Input: part model. Units: mm. Frame: model coordinates. A direction names the side the tool comes from. Give positions to 0.01 mm unless a question says otherwise; leave off trailing zeros. Write each loop counter-clockwise with the first axis right and the second up, starting at its lowest first coordinate (ties: lowest second). Pieces come first, ordered by that corner, then holes. Notation, with made-up numbers: (41, 50) -> (90, 50) arc R28 cw to (90, 73) -> close; hole circle Ø2 at (49.25, 57.5). An arc over 180 degrees is marked (long way). Answer as a JSON object with one key per item and string values. Group by question number.
Autodesk Inventor part; units mm, degrees
ref_plane "YZ Plane" through (0, 0, 0) normal (1, 0, 0) x (0, 1, 0)
ref_plane "XZ Plane" through (0, 0, 0) normal (0, 1, 0) x (-1, 0, 0)
ref_plane "XY Plane" through (0, 0, 0) normal (0, 0, 1) x (1, 0, 0)
sketch "Sketch1" plane through (0, 0, 0) normal (0, 0, 1) x (1, 0, 0)
  line L0 (0, 0) -> (0, 13.5)
  line L1 (0, 13.5) -> (36, 13.5)
  line L2 (36, 13.5) -> (36, 4.4)
  line L3 (36, 4.4) -> (40.4, 4.4)
  line L4 (40.4, 4.4) -> (40.4, 0)
  line L5 (40.4, 0) -> (0, 0)
  line L6 (0, 0) -> (68.0723, 0)
  dimension "d0" = 27
  dimension "d1" = 36
  dimension "d2" = 8.8
  dimension "d3" = 4.4
revolve "Revolution1" add sketch "Sketch1" angle 360 about axis through (0, 0, 0) along (1, 0, 0)
sketch "Sketch2" plane through (40.4, 0, 0) normal (1, 0, 0) x (0, 0, -1)
  circle A0 centre (0, 0) radius 4.4
  circle A1 centre (0, 0) radius 2.05
  dimension "d5" = 4.1
extrude "Extrusion1" add sketch "Sketch2" along normal blind 11 contours A1
sketch "Sketch3" plane through (36, 0, 0) normal (1, 0, 0) x (0, 0, -1)
  circle A0 centre (0, 0) radius 4.4
  circle A1 centre (0, 10) radius 1.5
  circle A2 centre (0, -10) radius 1.5
  dimension "d8" = 3
  dimension "d9" = 3
  dimension "d10" = 20
  dimension "d11" = 10
extrude "Extrusion2" cut sketch "Sketch3" against normal blind 5 contours A1 | A2
properties part number "Motor Sensor"
1. Section D-D (y = -10.75). Return the cut outline in (x, z), plus the area to 3 significant figures.
2. Mould query, pull axis Y, two halves, no side actions, for faces 1 (the face through (40.4, 2, -1)), 2 (the face through (38.231, 4.197, 1.322)), 3 (the face through (33.535, 8.536, 0.325)). Classes: pulls with the +Y half, pulls with the -Y half, needs draft (parallel to the pull), parting line crosses it, or undercut.
3. Contact query for flat-ended pins moving along their axis: pin 1 Ø1.5 at (x, y) = (14.5, 6.5) entering from -Z; pin 2 Ø8 at (x, y) = (23, -8.5) entering from -Z; pin 3 Ø6 at (x, y) = (8.5, -7) entering from +Z; pin 4 Ø10 at (x, y) = (21, -1) entering from +Z. Output: stop coordinate, or through.
4. Section C-C (x = 21). Return the cut outline in (y, z), plus the area to 3 significant figures.
5. Section B-B (z = 0). Return the cut outline in (x, y), plus the area to 3 significant figures.
6. Reachability of faces 4 (the face through (51.4, 0, 0)), 5 (the face through (31, 10, 0)) from +Z, -Z, +X, -X, +Y, -Y: full face, straight path, thin tool, end or side. Return the list, or none.
7. Line query: line 1 (X direction, y = -8.5, z = 7.5); line 2 (Z direction, x = 23, y = 0.5); line 3 (X direction, y = -2.75, z = -0.5). Output: solid intervals per line, ascending.
8. Section A-A (y = 0). Return the cut outline in (x, z).
Working result:
{
 "1": {"outline": "(0, -8.17) -> (36, -8.17) -> (36, -1.3) -> (31, -1.3) -> (31, 1.3) -> (36, 1.3) -> (36, 8.17) -> (0, 8.17) -> close", "area": "575 mm^2"},
 "2": {"face 1": "needs draft", "face 2": "parting line crosses it", "face 3": "undercut"},
 "3": {"pin 1": "stops at z = -12.21", "pin 2": "stops at z = -12.73", "pin 3": "stops at z = 12.89", "pin 4": "stops at z = 13.5"},
 "4": {"outline": "circle Ø27 at (0, 0)", "area": "573 mm^2"},
 "5": {"outline": "(0, -13.5) -> (36, -13.5) -> (36, -11.5) -> (31, -11.5) -> (31, -8.5) -> (36, -8.5) -> (36, -4.4) -> (40.4, -4.4) -> (40.4, -2.05) -> (51.4, -2.05) -> (51.4, 2.05) -> (40.4, 2.05) -> (40.4, 4.4) -> (36, 4.4) -> (36, 8.5) -> (31, 8.5) -> (31, 11.5) -> (36, 11.5) -> (36, 13.5) -> (0, 13.5) -> close", "area": "1,030 mm^2"},
 "6": {"face 4": "+Z, -Z, +X, +Y, -Y", "face 5": "+X"},
 "7": {"line 1": "x = 0 to 36", "line 2": "z = -13.49 to 13.49", "line 3": "x = 0 to 40.4"},
 "8": {"outline": "(0, -13.5) -> (36, -13.5) -> (36, -4.4) -> (40.4, -4.4) -> (40.4, -2.05) -> (51.4, -2.05) -> (51.4, 2.05) -> (40.4, 2.05) -> (40.4, 4.4) -> (36, 4.4) -> (36, 13.5) -> (0, 13.5) -> close"}
}
